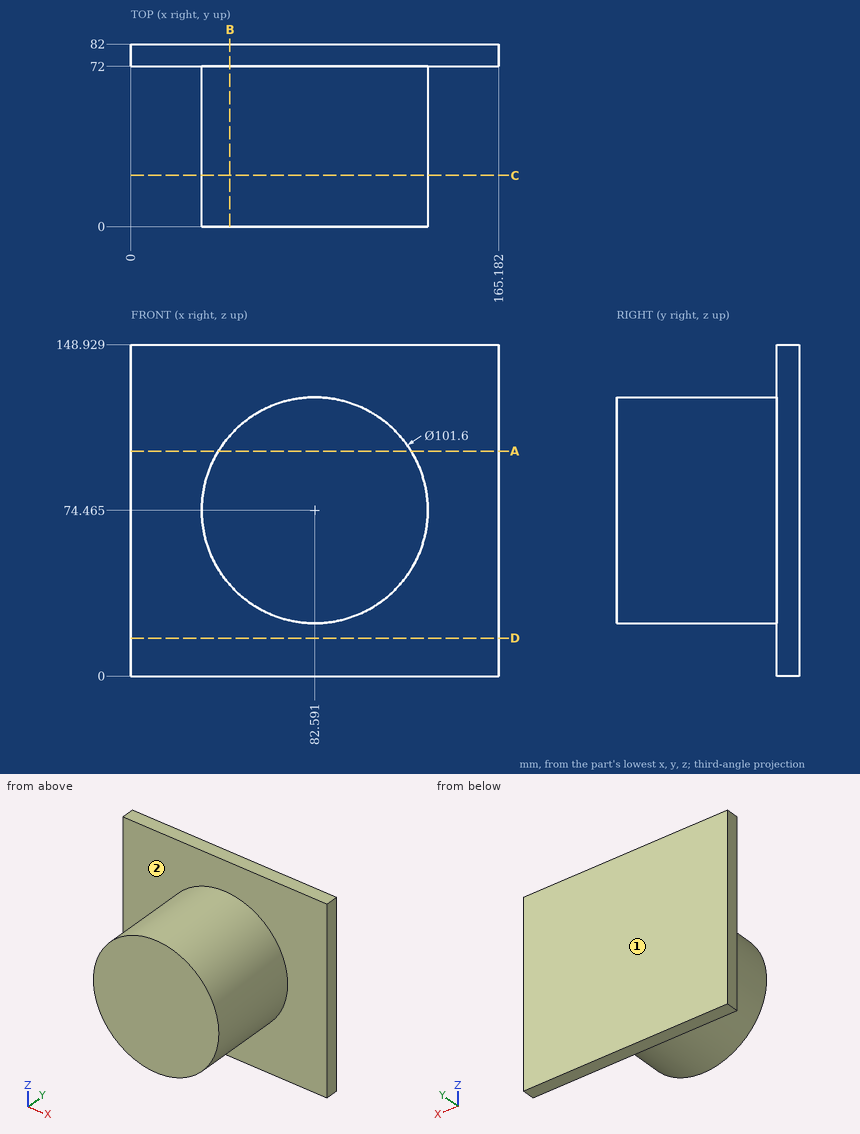
The drawing under review shows one solid part. Ordinate dimensions are in mm from its lowest x, y, z. A direction names the side the tool comes from. Give positions to 0.01 mm unless a question says otherwise; leave off trailing zeros. Write each loop counter-clockwise with the first axis right and the second up, starting at its lowest first coordinate (ties: lowest second). Pieces come first, ordered by that corner, then holes. Notation, with made-up numbers: (88, 33.25) -> (122, 33.25) arc R19 ccw to (122, 52.25) -> close; hole circle Ø3 at (71.25, 56.5). An arc over 180 degrees is marked (long way). Use CSV: the item, a comma, the result in double quotes.
Q1. To check wall thickness, follow probe 1 along Y at (x, z) = (9, 102); probe 2 along X at (y, z) = (65.5, 104); probe 3 along Z at (x, y) = (95.5, 33.5). State the ranges of each line that lie inside material, in increasing order. Write a range as [from, to].
Conclusion:
probe 1,"[72, 82]"
probe 2,"[41.26, 123.92]"
probe 3,"[25.33, 123.6]"
Q2. For P1, Ø6, axis at x = 92.5, y = 27.5, coming from the +Z side; P2, Ø10, axis at y = 36.5, z = 115, coming from the -X side; P3, Ø6, axis at y = 9, z = 110, coming from the +X side (1 decimal), all flat-tipped, find the tip position at first contact; note any pin that passes through.
Conclusion:
P1,"z = 124.79"
P2,"x = 46.29"
P3,"x = 121.6"
Q3. Take a section at D-D, the plane z = 17. Write out the cut boundary in (x, y).
Conclusion:
outline,"(0, 72) -> (165.18, 72) -> (165.18, 82) -> (0, 82) -> close"
Q4. Take a section at B-B, the plane x = 44.5. Write out the cut boundary in (y, z), then the cut area to 3 significant figures.
Conclusion:
outline,"(0, 40.85) -> (72, 40.85) -> (72, 0) -> (82, 0) -> (82, 148.93) -> (72, 148.93) -> (72, 108.08) -> (0, 108.08) -> close"
area,"6,330 mm2"
Q5. Take a section at A-A, the plane z = 101. Write out the cut boundary in (x, y), then the cut area to 3 significant figures.
Conclusion:
outline,"(0, 72) -> (39.27, 72) -> (39.27, 0) -> (125.91, 0) -> (125.91, 72) -> (165.18, 72) -> (165.18, 82) -> (0, 82) -> close"
area,"7,890 mm2"
Q6. Take a section at C-C, the plane y = 23. Write out the cut boundary in (x, z) (1 decimal).
Conclusion:
outline,"circle Ø101.6 at (82.6, 74.5)"
Q7. Tool access review of the marked faces 1 and 2: name each direction out of +Z, -Z, +X, -X, +Y, -Y from which nothing blocks a thin tool from reaching the whole face with its end or side.
Conclusion:
face 1,"+Z, -Z, +X, -X, +Y"
face 2,"-Y"
